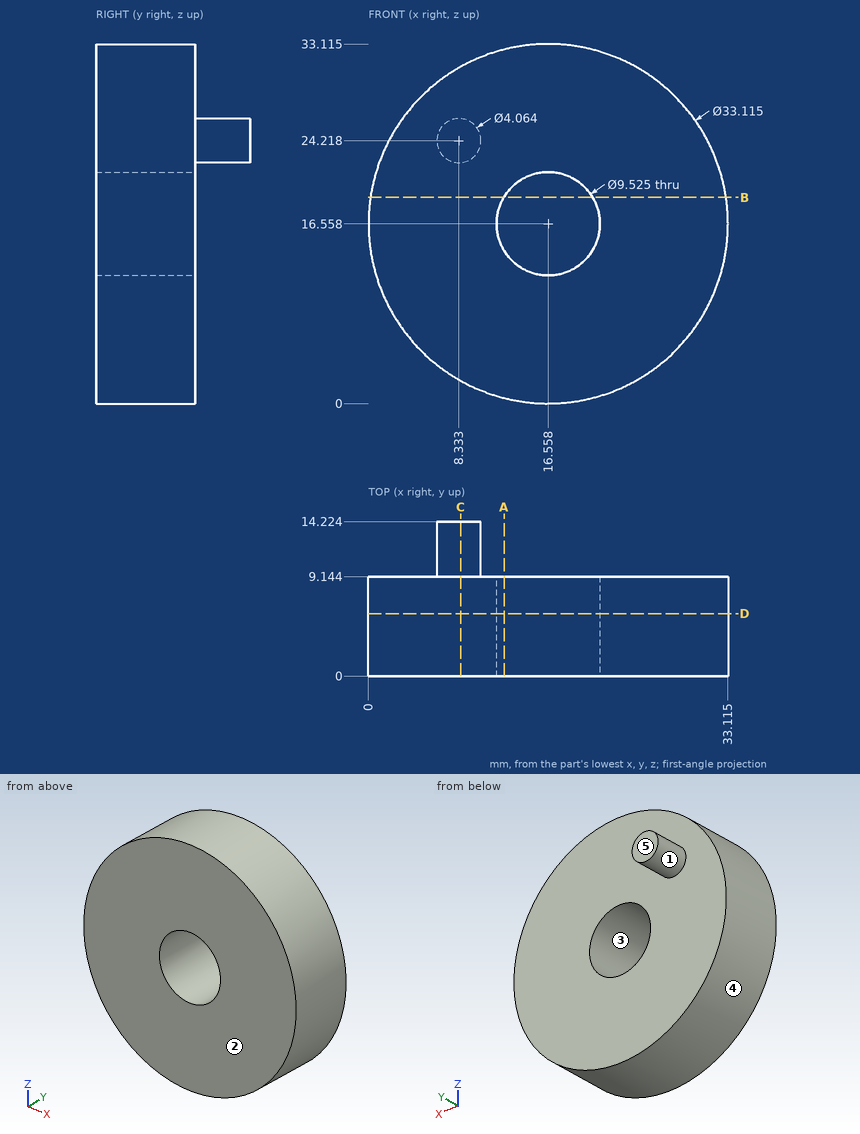
Input: dimensioned drawing with shaded views. Units: mm. Origin: part minimum x, y, z. A direction names the side the tool comes from. Round coordinates to 2 decimals unless told otherwise and drop trailing zeros. Order: outer loops, then holes, each group sorted by start corner. A loop starts at its lowest first (then second) coordinate and runs counter-clockwise, first axis right, second up. Notation, with made-up numbers: (-17.5, 42) -> (16.5, 42) arc R8 cw to (16.5, 51) -> close; hole circle Ø2 at (55.25, 73.25). An arc over 180 degrees is marked (long way). One line per item, written item: value. Start each with the question number.
Q1. Draft query along X for the marked faces 3, 4 and 5. Return one class per face: pulls with the +X half, pulls with the -X half, needs draft (parallel to the pull), parting line crosses it, or undercut.
Q2. Section query D-D (y = 5.75). Return the cut outline in (x, z) (1 decimal).
Q3. Section query A-A (x = 12.5). Return the cut outline in (y, z) (1 decimal), plus the area to 3 significant figures.
Q4. Material intervals for probe 1 along Y at (x, z) = (10.5, 24.5); probe 2 along Z at (x, y) = (19, 2) (1 decimal); probe 3 along X at (y, z) = (3, 18.5) (1 decimal), sorted ascending.
Q5. Section query C-C (x = 8.5). Return the cut outline in (y, z), plus the area to 3 significant figures.
Q6. Section query B-B (z = 19). Return the cut outline in (x, y), plus the area to 3 significant figures.
Q7. Access query for the marked faces 1 and 2. Directions: +Z, -Z, +X, -X, +Y, -Y. A direction counts if a zero-diameter tool reaches every point of the face in a straight line with its end or side. Return the directions, or none.
Q8. Pin query (flat end, axial travel): pin 1 (5 mm diameter, centred on x = 4, z = 11, fed in from +Y); pin 2 (4 mm diameter, centred on x = 6, z = 21.5, fed in from +Y); pin 3 (1 mm diameter, centred on x = 22, y = 9, fed in from -Z) (1 decimal); pin 4 (1.5 mm diameter, centred on y = 2.5, z = 4, fed in from -X). Return the tip coordinate at first contact, or that it passes through.
Findings below:
1. face 3: undercut
1. face 4: parting line crosses it
1. face 5: needs draft
2. outline: circle Ø33.1 at (16.6, 16.6); hole circle Ø9.5 at (16.6, 16.6)
3. outline: (0, 0.5) -> (9.1, 0.5) -> (9.1, 14.1) -> (0, 14.1) -> close; (0, 19.1) -> (9.1, 19.1) -> (9.1, 32.6) -> (0, 32.6) -> close
3. area: 248 mm²
4. probe 1: 0 to 9.14
4. probe 2: 0.2 to 12.5, 20.6 to 32.9
4. probe 3: 0.1 to 12.2, 20.9 to 33
5. outline: (0, 2.09) -> (9.14, 2.09) -> (9.14, 22.19) -> (14.22, 22.19) -> (14.22, 26.24) -> (9.14, 26.24) -> (9.14, 31.02) -> (0, 31.02) -> close
5. area: 285 mm²
6. outline: (0.18, 0) -> (12.47, 0) -> (12.47, 9.14) -> (0.18, 9.14) -> close; (20.65, 0) -> (32.93, 0) -> (32.93, 9.14) -> (20.65, 9.14) -> close
6. area: 225 mm²
7. face 1: +Y
7. face 2: +Z, -Z, +X, -X, -Y
8. pin 1: y = 9.14
8. pin 2: y = 14.22
8. pin 3: z = 0.8
8. pin 4: x = 4.95
